Could you check a few things on this model? Use its own coordinates, in mm. A direction names the side the tool comes from. Give positions to 0.01 mm unless a question says otherwise; leave off trailing zeros. Loops run counter-clockwise (first coordinate to the right, second up) from the corner with the lowest first, then second, coordinate; pieces in that order, holes last. Notation, with made-up numbers: (-19, 37.5) - (9, 37.5) arc R24 cw to (9, 51.5) - close; hole circle Ø3 at (80, 24). An arc over 180 degrees is marked (long way). Write each question's results on one line, items separated by ' | '. Start each with the question number.
1) I'm going to push flat-ended pins straight in: pin 1 (10 mm diameter, centred on y = 20.5, z = 8.5, fed in from +X); pin 2 (6 mm diameter, centred on x = -6.5, y = 5, fed in from +Z); pin 3 (4 mm diameter, centred on x = 0, z = -0.5, fed in from +Y). Where does each tip first touch, or does it pass through?
2) I want a section at A-A, the plane x = 0. Write out the boundary of the cut face in (y, z) (3 decimals), and give its area (3 significant figures).
3) I want a section at D-D, the plane y = 17.25. Write out the boundary of the cut face in (x, z) (3 decimals).
4) I want a section at B-B, the plane z = 0. Write out the boundary of the cut face in (x, y) (3 decimals), and give its area (3 significant figures).
5) On a 3-axis mill with a long thin cutter (end or side, diameter ignored), from which of +Z, -Z, +X, -X, +Y, -Y can I reach the whole of each face in a straight line? I mean faces 4 (the face through (-3, 25.4, -3)), 5 (the face through (0, 13.4, -8)). Say none if no direction works.
6) If I drill on probe 1 along Z at (x, y) = (0, 14.25) (3 decimals); probe 2 along Z at (x, y) = (0, 11.75) (3 decimals); probe 3 along X at (y, z) = (15.5, 3), over which ranges is the centre line in solid material (lowest first)? Write a range as [from, to].
7) I want a section at C-C, the plane y = 12.75. Write out the boundary of the cut face in (x, z) (3 decimals).
8) If we mould it in two halves opening along X, with no side actions, what happens to faces 1 (the face through (-2.75, 12.52, 12.4)), 2 (the face through (0, 0, 0)), 3 (the face through (0.67, 19.48, -9.18))? For each: +X half, -X half, draft (parallel to the pull), parting line (faces both ways), or undercut.
from build123d import *

# Parameters (mm, degrees)
SKETCH1_R           = 12.7
BOSS_EXTRUDE1_DEPTH = 25.4
SKETCH2_R           = 4.075
CUT_EXTRUDE1_DEPTH  = 19.05
SKETCH3_R           = 1.25
CUT_EXTRUDE2_DEPTH  = 12


with BuildPart() as part:
    # Sketch1 → Boss-Extrude1 (new body)
    with BuildSketch(Plane(origin=(0, 0, 0), x_dir=(1, 0, 0), z_dir=(0, 1, 0))):
        Circle(SKETCH1_R)
    extrude(amount=BOSS_EXTRUDE1_DEPTH)

    # Sketch2 → Cut-Extrude1 (cut)
    with BuildSketch(Plane(origin=(0, 25.4, 0), x_dir=(1, 0, 0), z_dir=(0, 1, 0))):
        Circle(SKETCH2_R)
    extrude(amount=-CUT_EXTRUDE1_DEPTH, mode=Mode.SUBTRACT)

    # Sketch3 → Cut-Extrude2 (cut)
    with BuildSketch(Plane(origin=(0, 25.4, 0), x_dir=(1, 0, 0), z_dir=(0, 1, 0))):
        with Locations((6.899904191, -1.930944627)):
            Circle(SKETCH3_R)
        with Locations((-5.25875141, -2.878464627)):
            Circle(SKETCH3_R)
        with Locations((0, 8.125)):
            Circle(SKETCH3_R)
    extrude(amount=-CUT_EXTRUDE2_DEPTH, mode=Mode.SUBTRACT)


solid = part.part
Answers:
1) pin 1: stops at x = 12.21 | pin 2: stops at z = 12.21 | pin 3: stops at y = 6.35
2) outline: (0, -12.7) - (25.4, -12.7) - (25.4, -9.375) - (13.4, -9.375) - (13.4, -6.875) - (25.4, -6.875) - (25.4, -4.075) - (6.35, -4.075) - (6.35, 4.075) - (25.4, 4.075) - (25.4, 12.7) - (0, 12.7) - close | area: 460 mm2
3) outline: circle Ø25.4 at (0, 0); hole circle Ø2.5 at (-5.259, 2.878); hole circle Ø8.15 at (0, 0); hole circle Ø2.5 at (0, -8.125); hole circle Ø2.5 at (6.9, 1.931)
4) outline: (-12.7, 0) - (12.7, 0) - (12.7, 25.4) - (4.075, 25.4) - (4.075, 6.35) - (-4.075, 6.35) - (-4.075, 25.4) - (-12.7, 25.4) - close | area: 490 mm2
5) face 4: +Z, -Z, +X, -X, +Y | face 5: +Y
6) probe 1: z = [-12.7, -9.375], [-6.875, -4.075], [4.075, 12.7] | probe 2: z = [-12.7, -4.075], [4.075, 12.7] | probe 3: x = [-12.34, -6.5], [-4.01, -2.76], [2.76, 6.25], [7.55, 12.34]
7) outline: circle Ø25.4 at (0, 0); hole circle Ø8.15 at (0, 0)
8) face 1: parting line | face 2: draft | face 3: undercut
